Geometry check sheet. Reference: drawing and pictorial views, mm from the part's lowest x, y, z. Round coordinates to 2 decimals unless told otherwise and drop trailing zeros. Loops run counter-clockwise (first coordinate to the right, second up) from the corner with the lowest first, then second, coordinate; pieces in that order, holes last. Notation, with made-up numbers: (81.25, 19.25) -> (124.25, 19.25) arc R19 cw to (124.25, 26.25) -> close; hole circle Ø5 at (-12.5, 14). An arc over 180 degrees is marked (long way). Use one line per item in the form item = value. Start each with the question number.
(1) Sectioned sample at C-C (y = 2.5). Record the cut outline in (x, z), and give its area (3 significant figures).
(2) Go/stop test with a flat-tipped pin: pin 1 (1.5 mm diameter, centred on y = 3.5, z = 98, fed in from +X). Record where the tip stops, or that it passes through.
(3) Material ranges on probe 1 along Z at (x, y) = (30, 1.45); probe 2 along X at (y, z) = (1.45, 31); probe 3 along X at (y, z) = (2.75, 97), recorded low to high. Write a range as [from, to].
(4) Sectioned sample at D-D (x = 12). Record the cut outline in (y, z), and give its area (3 significant figures).
(5) Sectioned sample at A-A (z = 31). Record the cut outline in (x, y), and give its area (3 significant figures).
(6) Sectioned sample at B-B (x = 30). Record the cut outline in (y, z), and give its area (3 significant figures).
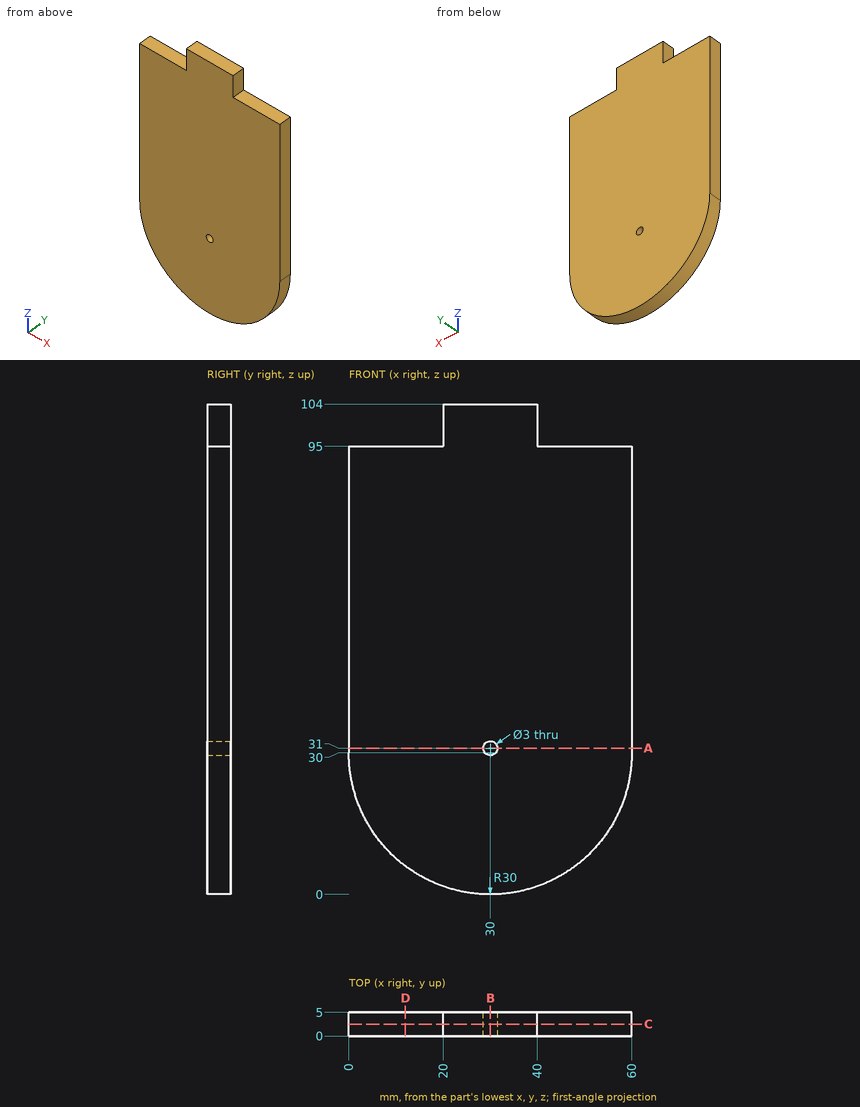
Checks:
q1.outline = (0, 30) arc R30 ccw to (60, 30) -> (60, 95) -> (40, 95) -> (40, 104) -> (20, 104) -> (20, 95) -> (0, 95) -> close; hole circle Ø3 at (30, 31)
q1.area = 5,490 mm2
q2.pin_1 = 40
q3.probe_1 = [0, 29.5], [32.5, 104]
q3.probe_2 = [0, 28.5], [31.5, 60]
q3.probe_3 = [20, 40]
q4.outline = (0, 6) -> (5, 6) -> (5, 95) -> (0, 95) -> close
q4.area = 445 mm2
q5.outline = (0, 0) -> (28.5, 0) -> (28.5, 5) -> (0, 5) -> close; (31.5, 0) -> (60, 0) -> (60, 5) -> (31.5, 5) -> close
q5.area = 285 mm2
q6.outline = (0, 0) -> (5, 0) -> (5, 29.5) -> (0, 29.5) -> close; (0, 32.5) -> (5, 32.5) -> (5, 104) -> (0, 104) -> close
q6.area = 505 mm2
